from build123d import *

# Parameters (mm, degrees)
IZIM1_W                     = 54
IZIM1_H                     = 3.5
Y_KSEKLIK_EKSTR_ZYON1_START = -30
Y_KSEKLIK_EKSTR_ZYON1_DEPTH = 10
RADYUS1_R                   = 1


with BuildPart() as part:
    # Çizim1 → Döndür1 (revolve)
    with BuildSketch(Plane.XY, mode=Mode.PRIVATE) as d_nd_r1_sk:
        with Locations((27, 1.75)):
            Rectangle(IZIM1_W, IZIM1_H)
    revolve(d_nd_r1_sk.sketch.rotate(Axis((0, 0, 0), (1, 0, 0)), 90), axis=Axis((0, 0, 0), (1, 0, 0)))

    # Çizim2 → Yükseklik-Ekstrüzyon1 (add)
    with BuildSketch(Plane(origin=(54, 0, 0), x_dir=(0, 0, -1), z_dir=(1, 0, 0)).offset(Y_KSEKLIK_EKSTR_ZYON1_START)):
        with BuildLine():
            Line((-1.5, 5.22), (1.5, 5.22))
            Line((1.5, 5.22), (1.5, 3.16227766))
            ThreePointArc((1.5, 3.16227766), (0, 3.5), (-1.5, 3.16227766))
            Line((-1.5, 3.16227766), (-1.5, 5.22))
        make_face()
    extrude(amount=Y_KSEKLIK_EKSTR_ZYON1_DEPTH)

    # Radyus1
    radyus1_edges = [part.edges().sort_by_distance(p)[0] for p in [
        (54, 0, -3.5),
    ]]
    fillet(radyus1_edges, radius=RADYUS1_R)


solid = part.part
Source: CAD feature listing. Evaluate the final solid. Frame: model axes, mm. A direction names the side the tool comes from. Round coordinates to 2 decimals unless told otherwise and drop trailing zeros. Loops run counter-clockwise (first coordinate to the right, second up) from the corner with the lowest first, then second, coordinate; pieces in that order, holes last. Notation, with made-up numbers: (18.25, 6) - (69.25, 6) arc R9 cw to (69.25, 11) - close; hole circle Ø10 at (66, 7). An arc over 180 degrees is marked (long way). Write item = value, one per line. Start each with the question number.
(1) Set-up query: faces 1 (the face through (29, 4, 1.5)), 2 (the face through (54, 0, 0)), 3 (the face through (29, 4, -1.5)). Return all of +Z, -Z, +X, -X, +Y, -Y with unobstructed straight access to the full face (end or side cutting, diameter ignored); none if empty.
(2) Ray query, line 1 along X through (y, z) = (3.5, -0.5); line 2 along Z through (x, y) = (33.5, 4.5); line 3 along Z through (x, y) = (25, -0.25). Return the intervals inside material, ascending. Write a range as from..to.
(3) Section query A-A, the plane z = 0. Output: boundary loops of the cut face in (x, y).
(4) Pin query (flat end, axial travel): pin 1 (2.5 mm diameter, centred on x = 28.5, y = 4.5, fed in from +Z); pin 2 (0.6 mm diameter, centred on y = 4, z = 0.5, fed in from +X); pin 3 (1.6 mm diameter, centred on x = 30.5, y = 4, fed in from -Z). Return the tip coordinate at first contact, or that it passes through.
(5) Section query B-B, the plane x = 40. Output: boundary loops of the cut face in (y, z), plus the area to 3 significant figures.
Conclusion:
q1.face_1 = +Z, +X, -X, +Y
q1.face_2 = +Z, -Z, +X, +Y, -Y
q1.face_3 = -Z, +X, -X, +Y
q2.line_1 = 24..34
q2.line_2 = -1.5..1.5
q2.line_3 = -3.49..3.49
q3.outline = (0, -3.5) - (53, -3.5) arc R1 ccw to (54, -2.5) - (54, 2.5) arc R1 ccw to (53, 3.5) - (34, 3.5) - (34, 5.22) - (24, 5.22) - (24, 3.5) - (0, 3.5) - close
q4.pin_1 = 1.5
q4.pin_2 = 34
q4.pin_3 = -1.5
q5.outline = circle Ø7 at (0, 0)
q5.area = 38.5 mm2
